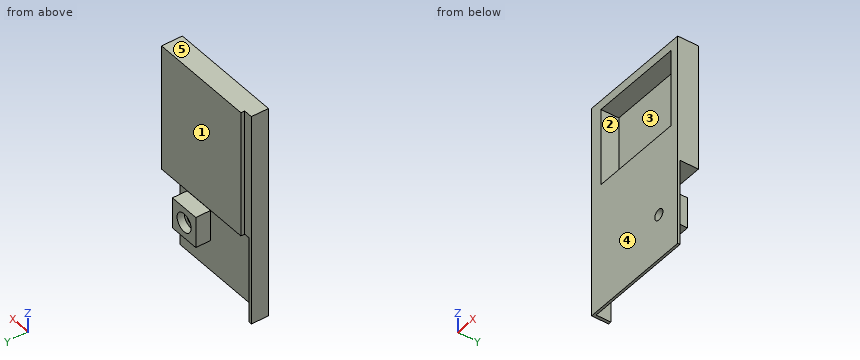
Autodesk Inventor part; units mm, degrees
ref_plane "YZ Plane" through (0, 0, 0) normal (1, 0, 0) x (0, 1, 0)
ref_plane "XZ Plane" through (0, 0, 0) normal (0, 1, 0) x (-1, 0, 0)
ref_plane "XY Plane" through (0, 0, 0) normal (0, 0, 1) x (1, 0, 0)
sketch "Sketch1" plane through (0, 0, 0) normal (0, 1, 0) x (-1, 0, 0)
  line L0 (19.325, 34.5) -> (-19.325, 34.5)
  line L1 (-19.325, 34.5) -> (-19.325, -34.5)
  line L2 (-19.325, -34.5) -> (19.325, -34.5)
  line L3 (19.325, -34.5) -> (19.325, 34.5)
  line L4 (19.325, 34.5) -> (-19.325, -34.5) construction
  line L5 (-19.325, 34.5) -> (19.325, -34.5) construction
  point P0 (0, 0)
  dimension "d0" = 38.65
  dimension "d1" = 69
extrude "Extrusion1" add sketch "Sketch1" along normal blind 5.5
sketch "Sketch3" plane through (0, 5.5, 0) normal (0, 1, 0) x (1, 0, 0)
  line L0 (19.325, -34.5) -> (19.325, 34.5)
  line L1 (19.325, -34.5) -> (-14.675, -34.5)
  line L2 (-14.675, -34.5) -> (-14.675, 6.5)
  line L3 (-14.675, 6.5) -> (19.325, 6.5)
  line L4 (19.325, 6.5) -> (19.325, -34.5)
  point P0 (0, 0)
  dimension "d4" = 34
  dimension "d5" = 41
extrude "Extrusion2" add sketch "Sketch3" along normal blind 1.2
sketch "Sketch4" plane through (-19.325, 0, -34.5) normal (-1, 0, 0) x (0, 0, 1)
  point P0 (34.5, 0)
sketch "Sketch5" plane through (0, 5.5, 0) normal (0, 1, 0) x (1, 0, 0)
  line L0 (19.325, 34.5) -> (-19.325, 34.5)
  line L1 (19.325, 34.5) -> (11.265, 34.5)
  circle A0 centre (11.265, 19.65) radius 2.4036
  line L2 (-14.675, -34.5) -> (19.325, -34.5)
  point P0 (0, 0)
  dimension "d20" = 8.06
  dimension "d21" = 54.15
hole "Hole1" at (11.265, 5.5, -19.65) direction (0, -1, 0) diameter 3.5 depth 10.5 tip angle 118 counterbore diameter 6 counterbore depth 2.3
sketch "Sketch6" plane through (0, 5.5, 0) normal (0, 1, 0) x (1, 0, 0)
  line L0 (19.325, -34.5) -> (19.325, 34.5)
  line L1 (19.325, 34.5) -> (-16.5957, 34.5)
  line L2 (-16.5957, 34.5) -> (-16.5957, 6.5)
  line L3 (-16.5957, 6.5) -> (19.325, 6.5)
  line L4 (19.325, 6.5) -> (19.325, 34.5)
  line L5 (16.265, 24.65) -> (6.265, 24.65)
  line L6 (6.265, 24.65) -> (6.265, 14.65)
  line L7 (6.265, 14.65) -> (16.265, 14.65)
  line L8 (16.265, 14.65) -> (16.265, 24.65)
  circle A0 centre (11.265, 19.65) radius 1.75
  line L9 (16.265, 24.65) -> (6.265, 14.65) construction
  line L10 (6.265, 24.65) -> (16.265, 14.65) construction
  point P0 (0, 0)
  point P1 (19.325, 6.5)
  dimension "d32" = 10
  dimension "d33" = 10
  dimension "d37" = 28
extrude "Extrusion3" cut sketch "Sketch6" against normal blind 4.75 contours L3 L2 L1 L0
sketch "Sketch7" plane through (0, 0, 0) normal (0, -1, 0) x (1, 0, 0)
  line L0 (-13.5462, 6.5334) -> (16.4538, 6.5334)
  line L1 (16.4538, 6.5334) -> (16.4538, 31.5334)
  line L2 (16.4538, 31.5334) -> (-13.5462, 31.5334)
  line L3 (-13.5462, 31.5334) -> (-13.5462, 6.5334)
  line L4 (-13.5462, 6.5334) -> (16.4538, 31.5334) construction
  line L5 (16.4538, 6.5334) -> (-13.5462, 31.5334) construction
  point P0 (0, 0)
  point P1 (1.4538, 19.0334)
  dimension "d40" = 30
  dimension "d41" = 25
extrude "Extrusion4" cut sketch "Sketch7" against normal blind 5.75
sketch "Sketch8" plane through (-19.325, 0, -34.5) normal (-1, 0, 0) x (0, 0, 1)
  line L0 (0, 0) -> (69, 0)
  line L1 (69, 0) -> (69, 5.5)
  line L2 (0, 0) -> (69, 0)
  line L3 (69, 0) -> (69, 5.5)
  line L4 (69, 5.5) -> (0, 5.5)
  line L5 (0, 5.5) -> (0, 0)
  point P0 (34.5, 0)
extrude "Extrusion5" cut sketch "Sketch8" against normal blind 1.75
properties part number "support_1"
Check sheet for the modelled part. Datum: model origin and axes. Units: mm. Face numbers are marked on the shaded views. A direction names the side the tool comes from. Round coordinates to 2 decimals unless told otherwise and drop trailing zeros. Write each loop counter-clockwise with the first axis right and the second up, starting at its lowest first coordinate (ties: lowest second). Pieces come first, ordered by that corner, then holes. Notation, with made-up numbers: (-33.75, 46) - (3.25, 46) arc R12 cw to (3.25, 59) - close; hole circle Ø1 at (0, 82.25). An arc over 180 degrees is marked (long way). Return JSON: item names as keys, results as strings.
Q1. Cross-section at C-C (x = -3.5). Record the boundary of the cut face in (y, z), then the cut area to 3 significant figures.
Returned:
{"outline": "(0, -34.5) - (0.75, -34.5) - (0.75, -6.5) - (6.7, -6.5) - (6.7, 34.5) - (0, 34.5) - (0, 31.53) - (5.75, 31.53) - (5.75, 6.53) - (0, 6.53) - close", "area": "152 mm²"}
Q2. Scan lines: L1, parallel to Z at x = 9, y = 1.25; L2, parallel to X at y = 4.3, z = -19.65 (3 decimals); L3, parallel to X at y = 1.3, z = -19.65 (3 decimals). Record each from-to range of solid material in increasing order. Write a range as from..to.
Returned:
{"L1": "z = -24.65..-14.65, -6.5..6.53, 31.53..34.5", "L2": "x = -17.575..-16.596, 6.265..8.265, 14.265..16.265", "L3": "x = -17.575..-16.596, 6.265..9.515, 13.015..16.265"}
Q3. Depth check by flat-ended pin: P1, Ø0.9, axis at x = -15.5, z = -3.5, coming from the +Y side; P2, Ø1.8, axis at x = 3, y = 2.5, coming from the -Z side. Enter the tip coordinate at first touch or a pass-through.
Returned:
{"P1": "stops at y = 5.5", "P2": "stops at z = -6.5"}
Q4. Cross-section at D-D (z = 19). Record the boundary of the cut face in (x, y) (3 decimals), then the cut area to 4 significant figures.
Returned:
{"outline": "(-17.575, 0) - (-13.546, 0) - (-13.546, 5.75) - (16.454, 5.75) - (16.454, 0) - (19.325, 0) - (19.325, 6.7) - (-14.675, 6.7) - (-14.675, 5.5) - (-17.575, 5.5) - close", "area": "71.25 mm²"}
Q5. Cross-section at B-B (y = 2.25). Record the boundary of the cut face in (x, z) (3 decimals).
Returned:
{"outline": "(-17.575, -34.5) - (-16.596, -34.5) - (-16.596, -6.5) - (19.325, -6.5) - (19.325, 34.5) - (-17.575, 34.5) - close; (6.265, -24.65) - (16.265, -24.65) - (16.265, -14.65) - (6.265, -14.65) - close; hole (-13.546, 6.533) - (16.454, 6.533) - (16.454, 31.533) - (-13.546, 31.533) - close; hole circle Ø3.5 at (11.265, -19.65)"}
Q6. Cross-section at A-A (z = -19.65). Record the boundary of the cut face in (x, y) (3 decimals).
Returned:
{"outline": "(-17.575, 0) - (9.515, 0) - (9.515, 3.2) - (8.265, 3.2) - (8.265, 5.5) - (6.265, 5.5) - (6.265, 0.75) - (-16.596, 0.75) - (-16.596, 5.5) - (-17.575, 5.5) - close; (13.015, 0) - (19.325, 0) - (19.325, 0.75) - (16.265, 0.75) - (16.265, 5.5) - (14.265, 5.5) - (14.265, 3.2) - (13.015, 3.2) - close"}
Q7. Draft check along Z on the marked faces 3, 4 and 5. Enter one of: released by +Z, released by -Z, zero draft, split by the parting line, or undercut.
Returned:
{"face 3": "undercut", "face 4": "zero draft", "face 5": "released by +Z"}
Q8. Access from +Z, -Z, +X, -X, +Y, -Y to the whole of each face (thin tool, end or side, straight path). Record for the marked faces 1 and 2.
Returned:
{"face 1": "+Z, -Z, +X, -X, +Y", "face 2": "-Y"}
